The model under review builds one solid part; all positions refer to its coordinate system, in mm. A direction names the side the tool comes from. Give positions to 0.01 mm unless a question says otherwise; leave off trailing zeros. Write each loop counter-clockwise with the first axis right and the second up, starting at its lowest first coordinate (ties: lowest second). Pieces come first, ordered by that corner, then holes. Notation, with made-up numbers: (56, -2) -> (101, -2) arc R18 ccw to (101, 25) -> close; hole circle Ø10 at (66.25, 58.5). An arc over 180 degrees is marked (long way). Use CSV: the item, a comma, the result in double quotes.
```python
from build123d import *

# Parameters (mm, degrees)
F1_DEPTH = 5
F2_W     = 34.4714387385
F2_H     = 10
F2_W_2   = 12.8498794511
F2_H_2   = 13.4021639824
F3_DEPTH = 5


# Not quite as in the source:
# - ends of sketch curves that miss each other by under 0.0002 mm in the source are joined
# - a feature names something its author has since deleted; it is built from what else it names


with BuildPart() as f1:
    # F0 (on Top) → F1 (new body)
    with BuildSketch(Plane.XY):
        with BuildLine():
            Line((0, 29.2999204248), (0, 0))
            Line((0, 0), (34.4714387385, 0))
            Line((34.4714387385, 0), (34.4714387385, 16.3473710418))
            ThreePointArc((34.4714387385, 16.3473710418), (32.5790927131, 15.1300794804), (32.2559916738, 17.3568210333))
            ThreePointArc((32.2559916738, 17.3568210333), (15.182844974, 14.8438668457), (5.7578901922, 29.2999210911))
            ThreePointArc((5.7578901922, 29.2999210911), (2.8789043427, 26.4210160822), (0, 29.2999204248))
        make_face()
        with BuildLine():
            ThreePointArc((5.7577396052, 29.3198639813), (2.8689325046, 32.1788074974), (0, 29.2999204248))
            ThreePointArc((0, 29.2999204248), (2.8789043427, 26.4210160822), (5.7578086853, 29.2999204248))
            ThreePointArc((5.7578086853, 29.2999204248), (5.7578117914, 29.3098925127), (5.7577396052, 29.3198639813))
        make_face()
        with BuildLine():
            ThreePointArc((32.2559916738, 17.3568210333), (32.5790927131, 15.1300794804), (34.4714387385, 16.3473710418))
            ThreePointArc((34.4714387385, 16.3473710418), (33.6883902233, 17.5646626032), (32.2559916738, 17.3568210333))
        make_face()
    extrude(amount=F1_DEPTH)

    # F2 (on face) → F3 (join)
    with BuildSketch(Plane.XY.offset(5)):
        with BuildLine():
            Line((0, 0), (34.4714387385, 0))
            Line((34.4714387385, 0), (34.4714387385, 16.3473710418))
            ThreePointArc((34.4714387385, 16.3473710418), (33.6883902233, 17.5646626032), (32.2559916738, 17.3568210333))
            ThreePointArc((32.2559916738, 17.3568210333), (15.182844974, 14.8438668457), (5.7578901922, 29.2999210911))
            ThreePointArc((5.7578901922, 29.2999210911), (5.757811792, 29.3098923335), (5.7577396052, 29.3198639813))
            ThreePointArc((5.7577396052, 29.3198639813), (2.8689325046, 32.1788074974), (0, 29.2999204248))
            Line((0, 29.2999204248), (0, 25.4882741719))
            Line((0, 25.4882741719), (0, 13.4021639824))
            Line((0, 13.4021639824), (0, 0))
        make_face()
        with Locations((17.2357193692, -5)):
            Rectangle(F2_W, F2_H)
        with Locations((-6.4249397255, 6.7010819912)):
            Rectangle(F2_W_2, F2_H_2)
    extrude(amount=-F3_DEPTH)


solid = f1.part
```
Q1. Machinability: for faces 5 (the flat face through (0, 21, 2)), 6 (the flat face through (-7, 0, 3)), 7 (the flat face through (34.471, 3, 2)), which of the approach directions +Z, -Z, +X, -X, +Y, -Y give a long, thin tool a straight path to every point of the face, cutting with its end or side? Answer none if there is none.
Derived:
face 5,"+Z, -Z, -X, +Y"
face 6,"+Z, -Z, -X, -Y"
face 7,"+Z, -Z, +X, +Y, -Y"
Q2. To check wall thickness, follow probe 1 along Y at (x, z) = (-0.5, 4.2); probe 2 along X at (y, z) = (-4, 2.45); probe 3 along X at (y, z) = (17, 0.8). State the ranges of each line that lie inside material, in increasing order.
Derived:
probe 1,"y = 0 to 13.4"
probe 2,"x = 0 to 34.47"
probe 3,"x = 0 to 11.68, 31.83 to 34.3"
Q3. Consider section C-C (x = 21.5). Write out the cut boundary in (y, z), then the cut area to 3 significant figures.
Derived:
outline,"(-10, 0) -> (13.43, 0) -> (13.43, 5) -> (-10, 5) -> close"
area,"117 mm2"
Q4. Consider section A-A (y = 14). Write out the cut boundary in (x, z).
Derived:
outline,"(0, 0) -> (17.53, 0) -> (17.53, 5) -> (0, 5) -> close; (25.99, 0) -> (34.47, 0) -> (34.47, 5) -> (25.99, 5) -> close"
Q5. The part is to be moulded in two halves that separate along X. For faces 1 (the cylindrical face through (33.708, 17.556, 2.465)), 2 (the flat face through (-12.85, 7, 3)), 3 (the flat face through (10, 7, 5)), 4 (the cylindrical face through (15.42, 14.74, 2.46)), say which applies: pulls with the +X half, pulls with the -X half, needs draft (parallel to the pull), parting line crosses it, or undercut.
Derived:
face 1,"undercut"
face 2,"pulls with the -X half"
face 3,"needs draft"
face 4,"undercut"
Q6. Consider section D-D (y = 27.5). Write out the cut boundary in (x, z).
Derived:
outline,"(0, 0) -> (5.87, 0) -> (5.87, 5) -> (0, 5) -> close"
Q7. Insertion check: pin 1 (1.5 mm diameter, centred on x = 6, z = 2, fed in from +Y); pin 2 (1 mm diameter, centred on y = 26.5, z = 2, fed in from +X); pin 3 (3 mm diameter, centred on x = 9, z = 3.5, fed in from +Y). Each pin has a flat end and moves straight along its axis. Give the tip position at first contact, or say it passes through.
Derived:
pin 1,"stops at y = 30.93"
pin 2,"stops at x = 6.13"
pin 3,"stops at y = 22.17"
